Input: part model. Units: mm. Frame: model coordinates. Face numbers are marked on the shaded views. A direction names the side the tool comes from. Give positions to 0.01 mm unless a question says otherwise; leave off trailing zeros. Loops run counter-clockwise (first coordinate to the right, second up) from the corner with the lowest first, then second, coordinate; pieces in that order, holes last. Notation, with made-up numbers: M 16,82 L 75,82 A30 cw 75,121 Z; hole C 64.25,-38 d5. An arc over 180 degrees is marked long. Answer as a JSON object with one key per item and string values. Group by question number.
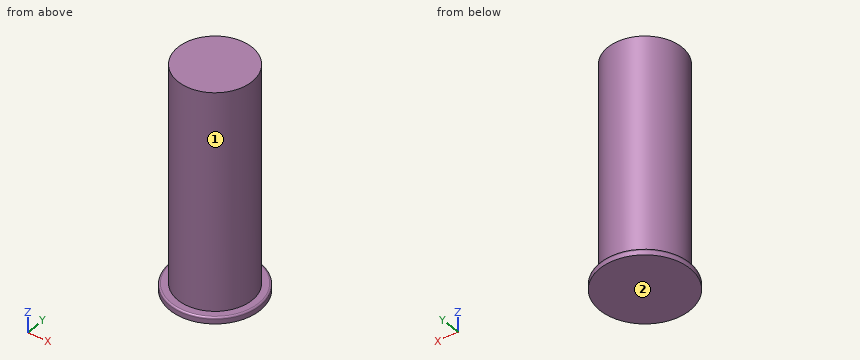
```python
from build123d import *

# Parameters (mm, degrees)
F0_R     = 11.5
F1_DEPTH = 70
F0_R_2   = 14
F2_DEPTH = 2
F3_R     = 0.5


with BuildPart() as f1:
    # F0 (on Top) → F1 (new body)
    with BuildSketch(Plane.XY):
        Circle(F0_R)
    extrude(amount=F1_DEPTH)

    # F0 (on Top) → F2 (join)
    with BuildSketch(Plane.XY):
        Circle(F0_R_2)
        Circle(F0_R, mode=Mode.SUBTRACT)
    extrude(amount=F2_DEPTH)

    # F3
    f3_edges = [f1.edges().sort_by_distance(p)[0] for p in [
        (-14, 0, 2),
    ]]
    fillet(f3_edges, radius=F3_R)


solid = f1.part
```
1. Material intervals for L1, parallel to Y at x = -0.25, z = 16; L2, parallel to Z at x = -7.75, y = -11, sorted ascending.
2. Section A-A (y = 0). Output: boundary loops of the cut face in (x, z).
3. Reachability of the marked faces 1 and 2 from +Z, -Z, +X, -X, +Y, -Y: full face, straight path, thin tool, end or side. Return the list, or none.
4. First-contact query: P1, Ø5, axis at x = 2, z = 60, coming from the +Y side; P2, Ø4, axis at x = 9.5, z = 21.5, coming from the -Y side; P3, Ø5, axis at y = 7, z = 33, coming from the +X side. Flat tips, straight axial feed; report the tip coordinate or a pass-through.
5. Section C-C (z = 62). Output: boundary loops of the cut face in (x, y).
Geometry results:
{
 "1": {"L1": "-11.5 to 11.5", "L2": "0 to 2"},
 "2": {"outline": "M -14,0 L 14,0 L 14,1.5 A0.5 ccw 13.5,2 L 11.5,2 L 11.5,70 L -11.5,70 L -11.5,2 L -13.5,2 A0.5 ccw -14,1.5 Z"},
 "3": {"face 1": "+Z", "face 2": "-Z, +X, -X, +Y, -Y"},
 "4": {"P1": "y = 11.5", "P2": "y = -8.72", "P3": "x = 10.58"},
 "5": {"outline": "C 0,0 d23"}
}
